```python
from build123d import *

# Parameters (mm, degrees)
BOSS_EXTRUDE1_DEPTH = 5
SKETCH2_W           = 5
SKETCH2_H           = 85
BOSS_EXTRUDE3_DEPTH = 110
SKETCH2_3_W         = 20
SKETCH2_3_H         = 19
BOSS_EXTRUDE4_DEPTH = 25
SKETCH3_R           = 1.45
CUT_EXTRUDE1_DEPTH  = 5
SKETCH4_R           = 1.45
CUT_EXTRUDE2_DEPTH  = 5
SKETCH5_R           = 3
SKETCH5_R_2         = 1.45
CUT_EXTRUDE3_DEPTH  = 3.1
SKETCH5_2_R         = 1.45
CUT_EXTRUDE4_DEPTH  = 5
CUT_EXTRUDE5_START  = -5
SKETCH6_R           = 1.45
CUT_EXTRUDE5_DEPTH  = 5
SKETCH2_7_W         = 33.25
SKETCH2_7_H         = 19
BOSS_EXTRUDE6_DEPTH = 72.25


with BuildPart() as part:
    # Sketch1 → Boss-Extrude1 (new body)
    with BuildSketch(Plane(origin=(0, 0, 0), x_dir=(0, 1, 0), z_dir=(0, 0, 1))):
        Polygon((-42.5, 94.306537639), (-42.5, -115), (42.5, -115), (42.5, 94.306537639), (42.5, 115), (-42.5, 115), align=None)
    extrude(amount=BOSS_EXTRUDE1_DEPTH)

    # Sketch2 → Boss-Extrude3 (add)
    with BuildSketch(Plane.XY.offset(5)):
        with Locations((-112.5, 0)):
            Rectangle(SKETCH2_W, SKETCH2_H)
        with Locations((112.5, 0)):
            Rectangle(SKETCH2_W, SKETCH2_H)
    extrude(amount=BOSS_EXTRUDE3_DEPTH)

    # Sketch2<3> → Boss-Extrude4 (add)
    with BuildSketch(Plane.XY.offset(5)):
        with Locations((-61.55, 0)):
            Rectangle(SKETCH2_3_W, SKETCH2_3_H)
        with Locations((-33.85, 0)):
            Rectangle(SKETCH2_3_W, SKETCH2_3_H)
        with Locations((-6.15, 0)):
            Rectangle(SKETCH2_3_W, SKETCH2_3_H)
        with Locations((21.55, 0)):
            Rectangle(SKETCH2_3_W, SKETCH2_3_H)
    extrude(amount=BOSS_EXTRUDE4_DEPTH)

    # Sketch3 → Cut-Extrude1 (cut)
    with BuildSketch(Plane(origin=(-115, 0, 0), x_dir=(0, -1, 0), z_dir=(-1, 0, 0))):
        with Locations((-15, 102)):
            Circle(SKETCH3_R)
        with Locations((15, 102)):
            Circle(SKETCH3_R)
        with BuildLine():
            Line((-3.75, 105.75), (3.75, 105.75))
            ThreePointArc((3.75, 105.75), (7.5, 102), (3.75, 98.25))
            Line((3.75, 98.25), (-3.75, 98.25))
            ThreePointArc((-3.75, 98.25), (-7.5, 102), (-3.75, 105.75))
        make_face()
    extrude(amount=-CUT_EXTRUDE1_DEPTH, mode=Mode.SUBTRACT)

    # Sketch4 → Cut-Extrude2 (cut)
    with BuildSketch(Plane.XY.offset(5)):
        with Locations((-47.7, 0)):
            Circle(SKETCH4_R)
        with Locations((7.181418717, 0)):
            Circle(SKETCH4_R)
    extrude(amount=-CUT_EXTRUDE2_DEPTH, mode=Mode.SUBTRACT)

    # Sketch5 → Cut-Extrude3 (cut)
    # profile 1 of 2: a face of its own
    with BuildSketch(Plane.YZ.offset(115)):
        with Locations(Location((-38.75, 111.25, 0), (0, 0, 270))):
            Circle(SKETCH5_R)
        with Locations(Location((-38.75, 111.25, 0), (0, 0, 270))):
            Circle(SKETCH5_R_2, mode=Mode.SUBTRACT)
    # profile 2 of 2: a face of its own
    with BuildSketch(Plane.YZ.offset(115)):
        with Locations(Location((38.75, 111.25, 0), (0, 0, 270))):
            Circle(SKETCH5_R)
        with Locations(Location((38.75, 111.25, 0), (0, 0, 270))):
            Circle(SKETCH5_R_2, mode=Mode.SUBTRACT)
    extrude(amount=-CUT_EXTRUDE3_DEPTH, mode=Mode.SUBTRACT)

    # Sketch5<2> → Cut-Extrude4 (cut)
    with BuildSketch(Plane.YZ.offset(115)):
        with Locations(Location((-38.75, 111.25, 0), (0, 0, 270))):
            Circle(SKETCH5_2_R)
        with Locations(Location((38.75, 111.25, 0), (0, 0, 270))):
            Circle(SKETCH5_2_R)
    extrude(amount=-CUT_EXTRUDE4_DEPTH, mode=Mode.SUBTRACT)

    # Sketch6 → Cut-Extrude5 (cut)
    with BuildSketch(Plane(origin=(-115, 0, 0), x_dir=(0, -1, 0), z_dir=(-1, 0, 0)).offset(CUT_EXTRUDE5_START)):
        with Locations(Location((-38.75, 111.25, 0), (0, 0, 270))):
            Circle(SKETCH6_R)
        with Locations(Location((38.75, 111.25, 0), (0, 0, 270))):
            Circle(SKETCH6_R)
    extrude(amount=CUT_EXTRUDE5_DEPTH, mode=Mode.SUBTRACT)

    # Sketch2<7> → Boss-Extrude6 (add)
    with BuildSketch(Plane.XY.offset(5)):
        with Locations((-93.375, 0)):
            Rectangle(SKETCH2_7_W, SKETCH2_7_H)
    extrude(amount=BOSS_EXTRUDE6_DEPTH)


solid = part.part
```
Source: CAD feature listing. Evaluate the final solid. Frame: model axes, mm. A direction names the side the tool comes from. Coordinates: 2 decimals unless noted, no trailing zeros. Write each loop counter-clockwise with the first axis right and the second up, starting at its lowest first coordinate (ties: lowest second). Pieces come first, ordered by that corner, then holes. Notation, with made-up numbers: (-12.5, 78) - (3.5, 78) arc R22 ccw to (3.5, 103) - close; hole circle Ø10 at (22, -21.5). An arc over 180 degrees is marked (long way). Answer as a JSON object with one key per item and string values.
Q1. Set-up query: faces 4 (the cylindrical face through (113.47, 39.65, 108.39)), 5 (the flat face through (-16.15, 0, 17)), 6 (the flat face through (-6, -9.5, 17)), 7 (the cylindrical face through (-112.5, 7.5, 101.9)). Return all of +Z, -Z, +X, -X, +Y, -Y with unobstructed straight access to the full face (end or side cutting, diameter ignored); none if empty.
Ans:
{"face 4": "+X", "face 5": "+Z, +Y, -Y", "face 6": "+Z, -Y", "face 7": "-X"}
Q2. Material intervals for line 1 (Y direction, x = 113.8, z = 111.25); line 2 (Y direction, x = 111.3, z = 111.25); line 3 (X direction, y = 8, z = 13.5), sorted ascending. Write a range as [from, to].
Ans:
{"line 1": "y = [-42.5, -41.75], [-35.75, 35.75], [41.75, 42.5]", "line 2": "y = [-42.5, -40.2], [-37.3, 37.3], [40.2, 42.5]", "line 3": "x = [-115, -76.75], [-71.55, -51.55], [-43.85, -23.85], [-16.15, 3.85], [11.55, 31.55], [110, 115]"}
Q3. Section query C-C, the plane x = -91.5. Output: boundary loops of the cut face in (y, z), plus the area to 3 significant figures.
Ans:
{"outline": "(-42.5, 0) - (42.5, 0) - (42.5, 5) - (9.5, 5) - (9.5, 77.25) - (-9.5, 77.25) - (-9.5, 5) - (-42.5, 5) - close", "area": "1,800 mm2"}
Q4. Draft query along X for faces 1 (the flat face through (-113, 0, 105.75)), 2 (the flat face through (111.9, 37, 112)), 3 (the flat face through (-34, -9.5, 17)). Return one class per face: released by +X, released by -X, zero draft, split by the parting line, or undercut.
Ans:
{"face 1": "zero draft", "face 2": "released by +X", "face 3": "undercut"}
Q5. Section query D-D, the plane z = 69.5. Output: boundary loops of the cut face in (x, y), plus the area to 3 significant figures.
Ans:
{"outline": "(-115, -42.5) - (-110, -42.5) - (-110, -9.5) - (-76.75, -9.5) - (-76.75, 9.5) - (-110, 9.5) - (-110, 42.5) - (-115, 42.5) - close; (110, -42.5) - (115, -42.5) - (115, 42.5) - (110, 42.5) - close", "area": "1,480 mm2"}
Q6. Section query A-A, the plane z = 82. Output: boundary loops of the cut face in (x, y).
Ans:
{"outline": "(-115, -42.5) - (-110, -42.5) - (-110, 42.5) - (-115, 42.5) - close; (110, -42.5) - (115, -42.5) - (115, 42.5) - (110, 42.5) - close"}
Q7. First-contact query: pin 1 Ø12 at (x, y) = (-58, 14) entering from +Z; pin 2 Ø4 at (y, z) = (38.75, 111.25) entering from +X; pin 3 Ø6 at (x, y) = (48.5, -22) entering from +Z. Flat tips, straight axial feed; report the tip coordinate or a pass-through.
Ans:
{"pin 1": "stops at z = 30", "pin 2": "stops at x = 111.9", "pin 3": "stops at z = 5"}
Q8. Section query B-B, the plane y = -33.5. Output: boundary loops of the cut face in (x, z), plus the area to 3 significant figures.
Ans:
{"outline": "(-115, 0) - (115, 0) - (115, 115) - (110, 115) - (110, 5) - (-110, 5) - (-110, 115) - (-115, 115) - close", "area": "2,250 mm2"}
